from build123d import *

# Parameters (mm, degrees)
SKETCH2_W            = 25.4
SKETCH2_H            = 48.26
BOSS_EXTRUDE1_DEPTH  = 3.81
SKETCH5_W            = 12.7
SKETCH5_H            = 33.02
CUT_EXTRUDE2_DEPTH   = 51.481501562
SKETCH4_W            = 22.86
SKETCH4_H            = 40.64
BOSS_EXTRUDE3_DEPTH  = 3.81
CHAMFER1_SIZE        = 6.35
SKETCH9_W            = 7.62
SKETCH9_H            = 6.35
BOSS_EXTRUDE4_DEPTH  = 2.8575
M3_CLEARANCE_HOLE1_D = 3.3
CHAMFER2_SIZE        = 12.7
CUT_EXTRUDE3_START   = -15.5575
CUT_EXTRUDE3_DEPTH   = 5.715


# Read off the part's stored shape, not the designer's step: Cut-Extrude3
# Some blends are built 0.0001 mm under size
with BuildPart() as part:
    # Sketch2 → Boss-Extrude1 (new, symmetric)
    with BuildSketch(Plane(origin=(0, 0, 0), x_dir=(0, 0, -1), z_dir=(1, 0, 0))):
        with Locations((0, 24.13)):
            Rectangle(SKETCH2_W, SKETCH2_H)
    extrude(amount=BOSS_EXTRUDE1_DEPTH, both=True)

    # Sketch5 → Cut-Extrude2 (cut, through all)
    with BuildSketch(Plane(origin=(3.81, 0, 0), x_dir=(0, 0, -1), z_dir=(1, 0, 0))):
        with Locations((0, 22.86)):
            Rectangle(SKETCH5_W, SKETCH5_H)
    extrude(amount=-CUT_EXTRUDE2_DEPTH, mode=Mode.SUBTRACT)

    # Sketch4 → Boss-Extrude3 (add)
    with BuildSketch(Plane(origin=(0, 0, 0), x_dir=(1, 0, 0), z_dir=(0, 1, 0))):
        Rectangle(SKETCH4_W, SKETCH4_H)
    extrude(amount=BOSS_EXTRUDE3_DEPTH)

    # Chamfer1
    chamfer1_edges = [part.edges().sort_by_distance(p)[0] for p in [
        (0, 39.37, 6.35),
        (0, 39.37, -6.35),
    ]]
    chamfer(chamfer1_edges, length=CHAMFER1_SIZE - 0.0001)  # a hair under: the kernel refuses the full size

    # Sketch9 → Boss-Extrude4 (add, symmetric)
    with BuildSketch(Plane.XY):
        with Locations((0, 51.435)):
            Rectangle(SKETCH9_W, SKETCH9_H)
    extrude(amount=BOSS_EXTRUDE4_DEPTH, both=True)

    # M3 Clearance Hole1 (through all)
    with Locations(Plane(origin=(0, 0, -12.7), x_dir=(-1, 0, 0), z_dir=(0, 0, -1))):
        with Locations((0, 50.8)):
            Hole(M3_CLEARANCE_HOLE1_D / 2)

    # Chamfer2
    # the kernel refuses this chamfer: 12.7 mm, written as the material it takes off along each edge
    with BuildSketch(Plane(origin=(36.470373947, 48.26, -12.7), x_dir=(0, -0.9996219169112966, -0.0274958766105866), z_dir=(-1, 0, 0))) as chamfer2_piece_1_section:
        Polygon((CHAMFER2_SIZE * 0.999621916911, CHAMFER2_SIZE * 0.0274958766106), (-CHAMFER2_SIZE * 0.0274958766106, CHAMFER2_SIZE * 0.999621916911), (0, 0), align=None)
    chamfer2_piece_1 = extrude(amount=72.940747894, mode=Mode.PRIVATE)
    chamfer2_piece_1 = split(chamfer2_piece_1, bisect_by=Plane(origin=(0, 43.83103101, -2.8575), z_dir=(0, 0, -1)), keep=Keep.TOP, mode=Mode.PRIVATE)
    add(chamfer2_piece_1, mode=Mode.SUBTRACT)
    with BuildSketch(Plane(origin=(-36.470373947, 48.26, 12.7), x_dir=(0, 0.02749587661058674, -0.9996219169112966), z_dir=(1, 0, 0))) as chamfer2_piece_2_section:
        Polygon((CHAMFER2_SIZE * 0.999621916911, -CHAMFER2_SIZE * 0.0274958766106), (-CHAMFER2_SIZE * 0.0274958766106, -CHAMFER2_SIZE * 0.999621916911), (0, 0), align=None)
    chamfer2_piece_2 = extrude(amount=72.940747894, mode=Mode.PRIVATE)
    chamfer2_piece_2 = split(chamfer2_piece_2, bisect_by=Plane(origin=(0, 43.83103101, 2.8575), z_dir=(0, 0, 1)), keep=Keep.TOP, mode=Mode.PRIVATE)
    add(chamfer2_piece_2, mode=Mode.SUBTRACT)

    # Cut-Extrude3 outline → Cut-Extrude3 (cut)
    with BuildSketch(Plane.XY.offset(12.7).offset(CUT_EXTRUDE3_START)):
        with BuildLine():
            Line((-3.81, 54.61), (-3.81, 50.8))
            ThreePointArc((-3.81, 50.8), (-2.694076836, 53.494076836), (0, 54.61))
            Line((0, 54.61), (-3.81, 54.61))
        make_face()
        with BuildLine():
            Line((3.81, 54.61), (0, 54.61))
            ThreePointArc((0, 54.61), (2.694076836, 53.494076836), (3.81, 50.8))
            Line((3.81, 50.8), (3.81, 54.61))
        make_face()
    extrude(amount=CUT_EXTRUDE3_DEPTH, mode=Mode.SUBTRACT)


solid = part.part
The listing builds one solid part. Answer for the finished solid, in the listing's coordinates (mm). A direction names the side the tool comes from. Coordinates: 2 decimals unless noted, no trailing zeros. Order: outer loops, then holes, each group sorted by start corner. A loop starts at its lowest first (then second) coordinate and runs counter-clockwise, first axis right, second up. Notation, with made-up numbers: (-30, 82.25) -> (-14, 82.25) arc R35 ccw to (-14, 120.25) -> close; hole circle Ø1 at (56, 27). An arc over 180 degrees is marked (long way). Answer in a Markdown table with one row per item. Add a question column.
Item 1: Which of the six approach directions +Z, -Z, +X, -X, +Y, -Y give full straight-line access (tool end or side, diameter ignored) to faces 4 (the face through (3.81, 28, -8)), 5 (the face through (0.05, 36.24, -3.13)), 6 (the face through (0, 49, -2.858)), 7 (the face through (-3.81, 28, -8))?
Item 2: Find section B-B (z = 4). Write down the section's boundary in (x, y).
Item 3: Find section A-A (y = 14). Write down the section's boundary in (x, z).
Item 4: Each of these flat-tipped pins is pushed along its axis until it touches: P1, Ø1.5, axis at x = 3.5, z = -1, coming from the +Y side; P2, Ø7.5, axis at y = 24.5, z = 2, coming from the -X side; P3, Ø12, axis at x = -3, y = 12, coming from the -Z side; P4, Ø2.5, axis at x = -2, y = 49, coming from the +Z side. Where does it stop, or does it pass through?
Item 5: Determine the mould class of faces 1 (the face through (0, 0, 0)), 2 (the face through (0, 6.35, 0)), 3 (the face through (-11.43, 2, 0)) for opening direction Y: +Y half, -Y half, draft (parallel to the pull), parting line (faces both ways), or undercut.
Item 6: Find section D-D (x = -5.5). Write down the section's boundary in (y, z).
Item 7: Find the intervals of material crossed by L1, parallel to Z at x = 1.5, y = 11.5; L2, parallel to Y at x = 6.25, z = 7; L3, parallel to X at y = 10.5, z = 8.5, in increasing order. Write a range as from..to.
Item 8: Find section C-C (z = 8.5). Write down the section's boundary in (x, y), then the cut area to 3 significant figures.
Result set:
| question | item | result |
|---|---|---|
| 1 | face 4 | +Z, -Z, +X, +Y |
| 1 | face 5 | +X, -X |
| 1 | face 6 | -Z, +X, -X, +Y |
| 1 | face 7 | +Z, -Z, -X, +Y |
| 2 | outline | (-11.43, 0) -> (11.43, 0) -> (11.43, 3.81) -> (3.81, 3.81) -> (3.81, 6.35) -> (-3.81, 6.35) -> (-3.81, 3.81) -> (-11.43, 3.81) -> close; (-3.81, 35.37) -> (3.81, 35.37) -> (3.81, 44.26) -> (-3.81, 44.26) -> close |
| 3 | outline | (-3.81, -12.7) -> (3.81, -12.7) -> (3.81, -6.35) -> (-3.81, -6.35) -> close; (-3.81, 6.35) -> (3.81, 6.35) -> (3.81, 12.7) -> (-3.81, 12.7) -> close |
| 4 | P1 | stops at y = 53.44 |
| 4 | P2 | passes through |
| 4 | P3 | stops at z = -12.7 |
| 4 | P4 | stops at z = 2.86 |
| 5 | face 1 | -Y half |
| 5 | face 2 | undercut |
| 5 | face 3 | draft |
| 6 | outline | (0, -20.32) -> (3.81, -20.32) -> (3.81, 20.32) -> (0, 20.32) -> close |
| 7 | L1 | z = -12.7..-6.35, 6.35..12.7 |
| 7 | L2 | y = 0..3.81 |
| 7 | L3 | x = -3.81..3.81 |
| 8 | outline | (-11.43, 0) -> (11.43, 0) -> (11.43, 3.81) -> (3.81, 3.81) -> (3.81, 39.76) -> (-3.81, 39.76) -> (-3.81, 3.81) -> (-11.43, 3.81) -> close |
| 8 | area | 361 mm² |
